from build123d import *

# Parameters (mm, degrees)
BOSS_EXTRUDE1_DEPTH = 55
BOSS_EXTRUDE2_DEPTH = 2
SKETCH3_W           = 22.6
SKETCH3_H           = 10
CUT_EXTRUDE1_DEPTH  = 12
FILLET1_R           = 1
BOSS_EXTRUDE3_DEPTH = 5


with BuildPart() as part:
    # Sketch1 → Boss-Extrude1 (new body)
    with BuildSketch(Plane.XY):
        with BuildLine():
            Line((36.5, -14.5), (-36.5, -14.5))
            ThreePointArc((-36.5, -14.5), (-37.914213562, -13.914213562), (-38.5, -12.5))
            Line((-38.5, -12.5), (-38.5, 12.5))
            ThreePointArc((-38.5, 12.5), (-37.914213562, 13.914213562), (-36.5, 14.5))
            Line((-36.5, 14.5), (36.5, 14.5))
            ThreePointArc((36.5, 14.5), (37.914213562, 13.914213562), (38.5, 12.5))
            Line((38.5, 12.5), (38.5, -12.5))
            ThreePointArc((38.5, -12.5), (37.914213562, -13.914213562), (36.5, -14.5))
        make_face()
        with BuildLine():
            Line((-34.5, -12.5), (34.5, -12.5))
            ThreePointArc((34.5, -12.5), (35.914213562, -11.914213562), (36.5, -10.5))
            Line((36.5, -10.5), (36.5, 10.5))
            ThreePointArc((36.5, 10.5), (35.914213562, 11.914213562), (34.5, 12.5))
            Line((34.5, 12.5), (-34.5, 12.5))
            ThreePointArc((-34.5, 12.5), (-35.914213562, 11.914213562), (-36.5, 10.5))
            Line((-36.5, 10.5), (-36.5, -10.5))
            ThreePointArc((-36.5, -10.5), (-35.914213562, -11.914213562), (-34.5, -12.5))
        make_face(mode=Mode.SUBTRACT)
    extrude(amount=BOSS_EXTRUDE1_DEPTH)

    # Sketch2 → Boss-Extrude2 (add)
    with BuildSketch(Plane.XY.offset(55)):
        with BuildLine():
            Line((-36.5, -14.5), (36.5, -14.5))
            ThreePointArc((36.5, -14.5), (37.914213562, -13.914213562), (38.5, -12.5))
            Line((38.5, -12.5), (38.5, 12.5))
            ThreePointArc((38.5, 12.5), (37.914213562, 13.914213562), (36.5, 14.5))
            Line((36.5, 14.5), (-36.5, 14.5))
            ThreePointArc((-36.5, 14.5), (-37.914213562, 13.914213562), (-38.5, 12.5))
            Line((-38.5, 12.5), (-38.5, -12.5))
            ThreePointArc((-38.5, -12.5), (-37.914213562, -13.914213562), (-36.5, -14.5))
        make_face()
    extrude(amount=BOSS_EXTRUDE2_DEPTH)

    # Sketch3 → Cut-Extrude1 (cut)
    with BuildSketch(Plane.XY.offset(57)):
        with Locations((-20.033386602, 0)):
            Rectangle(SKETCH3_W, SKETCH3_H)
        with Locations((20.033386602, 0)):
            Rectangle(SKETCH3_W, SKETCH3_H)
    extrude(amount=-CUT_EXTRUDE1_DEPTH, mode=Mode.SUBTRACT)

    # Fillet1
    fillet1_edges = [part.edges().sort_by_distance(p)[0] for p in [
        (-37.914213562, -13.914213562, 57),
        (0, -14.5, 57),
        (37.914213562, -13.914213562, 57),
        (38.5, 0, 57),
        (37.914213562, 13.914213562, 57),
        (0, 14.5, 57),
        (-37.914213562, 13.914213562, 57),
        (-38.5, 0, 57),
    ]]
    fillet(fillet1_edges, radius=FILLET1_R)

    # Sketch4 → Boss-Extrude3 (add)
    with BuildSketch(Plane(origin=(0, 0, 0), x_dir=(-1, 0, 0), z_dir=(0, 0, -1))):
        with BuildLine():
            Line((38.5, -12.5), (38.5, 12.5))
            ThreePointArc((38.5, 12.5), (37.914213562, 13.914213562), (36.5, 14.5))
            Line((36.5, 14.5), (-36.5, 14.5))
            ThreePointArc((-36.5, 14.5), (-37.914213562, 13.914213562), (-38.5, 12.5))
            Line((-38.5, 12.5), (-38.5, -12.5))
            ThreePointArc((-38.5, -12.5), (-37.914213562, -13.914213562), (-36.5, -14.5))
            Line((-36.5, -14.5), (36.5, -14.5))
            ThreePointArc((36.5, -14.5), (37.914213562, -13.914213562), (38.5, -12.5))
        make_face()
        with BuildLine():
            Line((-34.5, -12.5), (34.5, -12.5))
            ThreePointArc((34.5, -12.5), (35.914213562, -11.914213562), (36.5, -10.5))
            Line((36.5, -10.5), (36.5, 10.5))
            ThreePointArc((36.5, 10.5), (35.914213562, 11.914213562), (34.5, 12.5))
            Line((34.5, 12.5), (-34.5, 12.5))
            ThreePointArc((-34.5, 12.5), (-35.914213562, 11.914213562), (-36.5, 10.5))
            Line((-36.5, 10.5), (-36.5, -10.5))
            ThreePointArc((-36.5, -10.5), (-35.914213562, -11.914213562), (-34.5, -12.5))
        make_face(mode=Mode.SUBTRACT)
    extrude(amount=BOSS_EXTRUDE3_DEPTH)


solid = part.part
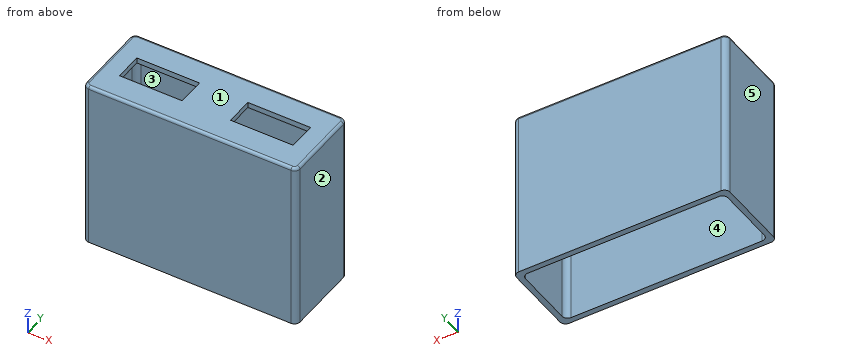
Can you work these out from the model? Positions are in its coordinate system, mm. Face numbers are marked on the shaded views. A direction names the side the tool comes from. Give positions to 0.01 mm unless a question says otherwise; leave off trailing zeros. Write each loop counter-clockwise with the first axis right and the second up, starting at its lowest first coordinate (ties: lowest second). Pieces come first, ordered by that corner, then holes. Notation, with made-up numbers: M 38.5,87 L 90.5,87 A20 ccw 90.5,123 Z; hole C 25.5,-16 d4. An arc over 180 degrees is marked long. Answer in a Markdown table with one row per item. Add a question column.
Item 1: Imagine slicing it at A-A, the plane y = 3.75. Write out the boundary of the cut face in (x, z).
Item 2: Imagine slicing it at B-B, the plane x = -11. Write out the boundary of the cut face in (y, z), plus the area to 3 significant figures.
Item 3: Please list where these lines run through material, in increasing order: L1, parallel to Y at x = 14, z = 26; L2, parallel to X at y = 5.25, z = 13; L3, parallel to Z at x = -23, y = 8.
Item 4: We'd pull the mould along X, two halves only. Please class the marked faces 1, 2 and 3: released by +X, released by -X, zero draft, split by the parting line, or undercut.
Item 5: Imagine slicing it at D-D, the plane y = -8.75. Write out the boundary of the cut face in (x, z).
Item 6: On a 3-axis mill with a long thin cutter (end or side, diameter ignored), from which of +Z, -Z, +X, -X, +Y, -Y can I reach the whole of each face in a straight line? I mean the marked faces 4 and 5. Say none if no direction works.
Item 7: For pin 1 Ø0.6 at (x, z) = (18, 56.5) entering from -Y; pin 2 Ø4 at (x, y) = (24, 6.5) entering from -Z, each with a flat end and sliding along its axis, tell me the tip position at first contact or that it passes through.
Item 8: Imagine slicing it at C-C, the plane z = 50.5. Write out the boundary of the cut face in (x, y), plus the area to 3 significant figures.
Evaluation:
| question | item | result |
|---|---|---|
| 1 | outline | M -38.5,-5 L -36.5,-5 L -36.5,55 L -31.33,55 L -31.33,57 L -37.5,57 A1 ccw -38.5,56 Z; M -8.73,55 L 8.73,55 L 8.73,57 L -8.73,57 Z; M 31.33,55 L 36.5,55 L 36.5,-5 L 38.5,-5 L 38.5,56 A1 ccw 37.5,57 L 31.33,57 Z |
| 2 | outline | M -14.5,-5 L -12.5,-5 L -12.5,55 L -5,55 L -5,57 L -13.5,57 A1 ccw -14.5,56 Z; M 5,55 L 12.5,55 L 12.5,-5 L 14.5,-5 L 14.5,56 A1 ccw 13.5,57 L 5,57 Z |
| 2 | area | 278 mm² |
| 3 | L1 | y = -14.5 to -12.5, 12.5 to 14.5 |
| 3 | L2 | x = -38.5 to -36.5, 36.5 to 38.5 |
| 3 | L3 | z = 55 to 57 |
| 4 | face 1 | zero draft |
| 4 | face 2 | released by +X |
| 4 | face 3 | undercut |
| 5 | outline | M -38.5,-5 L -36.5,-5 L -36.5,55 L 36.5,55 L 36.5,-5 L 38.5,-5 L 38.5,56 A1 ccw 37.5,57 L -37.5,57 A1 ccw -38.5,56 Z |
| 6 | face 4 | -Z |
| 6 | face 5 | +Z, -Z, -X, +Y, -Y |
| 7 | pin 1 | stops at y = -14.48 |
| 7 | pin 2 | stops at z = 55 |
| 8 | outline | M -38.5,-12.5 A2 ccw -36.5,-14.5 L 36.5,-14.5 A2 ccw 38.5,-12.5 L 38.5,12.5 A2 ccw 36.5,14.5 L -36.5,14.5 A2 ccw -38.5,12.5 Z; hole M -36.5,-10.5 A2 ccw -34.5,-12.5 L 34.5,-12.5 A2 ccw 36.5,-10.5 L 36.5,10.5 A2 ccw 34.5,12.5 L -34.5,12.5 A2 ccw -36.5,10.5 Z |
| 8 | area | 408 mm² |
